```python
from build123d import *

# Parameters (mm, degrees)
P_IDAT_VYSUNUT_M1_DEPTH = 30
P_IDAT_START            = -2
SKICA2_R                = 1.15
P_IDAT_VYSUNUT_M2_DEPTH = 3
P_IDAT_VYSUNUT_M3_DEPTH = 1


with BuildPart() as part:
    # Skica1 → Přidat vysunutím1 (new body)
    with BuildSketch(Plane(origin=(0, 0, 0), x_dir=(1, 0, 0), z_dir=(0, 1, 0))):
        Polygon((-5, 0), (5, 0), (5, 1.6), (4, 2.6), (4, 3), (5, 3), (5, 3.6), (6.2, 3.6), (6.2, -1), (-6.2, -1), (-6.2, 3.6), (-5, 3.6), (-5, 3), (-4, 3), (-4, 2.6), (-5, 1.6), align=None)
    p_idat_vysunut_m1 = extrude(amount=P_IDAT_VYSUNUT_M1_DEPTH)

    # Skica2 → Přidat vysunutím2 (add)
    with BuildSketch(Plane.XY.offset(P_IDAT_START)):
        with BuildLine():
            Line((-10.2, 17.5), (-10.6, 17.5))
            ThreePointArc((-10.6, 17.5), (-12.014213562, 16.914213562), (-12.6, 15.5))
            Line((-12.6, 15.5), (-12.6, 14.5))
            ThreePointArc((-12.6, 14.5), (-12.014213562, 13.085786438), (-10.6, 12.5))
            Line((-10.6, 12.5), (-10.2, 12.5))
            ThreePointArc((-10.2, 12.5), (-7.371572875, 11.328427125), (-6.2, 8.5))
            Line((-6.2, 8.5), (-6.2, 21.5))
            ThreePointArc((-6.2, 21.5), (-7.371572875, 18.671572875), (-10.2, 17.5))
        make_face()
        with Locations((-10.2, 15)):
            Circle(SKICA2_R, mode=Mode.SUBTRACT)
    p_idat_vysunut_m2 = extrude(amount=P_IDAT_VYSUNUT_M2_DEPTH)

    # Skica3 → Přidat vysunutím3 (add)
    with BuildSketch(Plane.XY.offset(1)):
        with BuildLine():
            Line((-6.2, 30), (6.2, 30))
            Line((6.2, 30), (6.2, 33))
            Line((6.2, 33), (5.959807907, 33))
            ThreePointArc((5.959807907, 33), (0.150662271, 32.3427273), (-5.364776224, 30.404140537))
            Line((-5.364776224, 30.404140537), (-6.2, 30))
        make_face()
    p_idat_vysunut_m3 = extrude(amount=-P_IDAT_VYSUNUT_M3_DEPTH)

    # Zrcadlit2: Přidat vysunutím1, Přidat vysunutím2, Přidat vysunutím3 across plane
    add(p_idat_vysunut_m1.mirror(Plane(origin=(6.2, 30, -3.6), x_dir=(0, 0, 1), z_dir=(-1, 0, 0))))
    add(p_idat_vysunut_m2.mirror(Plane(origin=(6.2, 30, -3.6), x_dir=(0, 0, 1), z_dir=(-1, 0, 0))))
    add(p_idat_vysunut_m3.mirror(Plane(origin=(6.2, 30, -3.6), x_dir=(0, 0, 1), z_dir=(-1, 0, 0))))


solid = part.part
```
Input: part model. Units: mm. Frame: model coordinates. A direction names the side the tool comes from. Coordinates: 2 decimals unless noted, no trailing zeros. Write each loop counter-clockwise with the first axis right and the second up, starting at its lowest first coordinate (ties: lowest second). Pieces come first, ordered by that corner, then holes.
1) Mould query, pull axis Y, two halves, no side actions, for faces 5 (the cylindrical face through (23.51, 14.3, -0.52)), 6 (the flat face through (17, 15, -3)), 7 (the flat face through (6, 30, -2)). Classes: pulls with the +Y half, pulls with the -Y half, needs draft (parallel to the pull), parting line crosses it, or undercut.
2) Section D-D on x = 0. Output: boundary loops of the cut face in (y, z).
3) Material intervals for line 1 along X through (y, z) = (21.5, -1.35); line 2 along Y through (x, z) = (-10.2, 0.3); line 3 along X through (y, z) = (5.5, -2.1), sorted ascending.
4) Section A-A on z = -1. State how many separate pieces and enclosed holes the cut face has, and give its area (3 significant figures).
5) Section B-B on y = 26. Output: boundary loops of the cut face in (x, z).
6) Pin query (flat end, axial travel): pin 1 Ø1 at (y, z) = (9.5, -2) entering from +X; pin 2 Ø0.5 at (y, z) = (17, -1) entering from -X; pin 3 Ø0.5 at (x, y) = (8, 14) entering from -Z. Return the tip coordinate at first contact, or that it passes through.
7) Set-up query: faces 1 (the flat face through (-4.5, 14.8, -3)), 2 (the flat face through (4.5, 14.8, -2.1)), 3 (the flat face through (21, 15, -2)), 4 (the flat face through (-6.2, 14.8, -2.3)). Return all of +Z, -Z, +X, -X, +Y, -Y with unobstructed straight access to the full face (end or side cutting, diameter ignored); none if empty.
Check result:
1. face 5: undercut
1. face 6: needs draft
1. face 7: pulls with the +Y half
2. outline: (0, 0) - (32.31, 0) - (32.31, 1) - (0, 1) - close
3. line 1: x = -6.2 to -5, 5 to 7.4, 17.4 to 18.6
3. line 2: y = 12.5 to 13.85, 16.15 to 17.5
3. line 3: x = -6.2 to -4.5, 4.5 to 7.9, 16.9 to 18.6
4. separate pieces: 3
4. enclosed holes: 2
4. area: 210 mm2
5. outline: (-6.2, -3.6) - (-5, -3.6) - (-5, -3) - (-4, -3) - (-4, -2.6) - (-5, -1.6) - (-5, 0) - (5, 0) - (5, -1.6) - (4, -2.6) - (4, -3) - (5, -3) - (5, -3.6) - (7.4, -3.6) - (7.4, -3) - (8.4, -3) - (8.4, -2.6) - (7.4, -1.6) - (7.4, 0) - (17.4, 0) - (17.4, -1.6) - (16.4, -2.6) - (16.4, -3) - (17.4, -3) - (17.4, -3.6) - (18.6, -3.6) - (18.6, 1) - (-6.2, 1) - close
6. pin 1: stops at x = 18.89
6. pin 2: stops at x = -12.16
6. pin 3: stops at z = -3
7. face 1: -Z, +Y, -Y
7. face 2: +Y, -Y
7. face 3: -Z, +X, +Y, -Y
7. face 4: -Z, -X
